from build123d import *

# Parameters (mm, degrees)
SKETCH1_W           = 230
SKETCH1_H           = 150
BOSS_EXTRUDE1_DEPTH = 6
SKETCH2_W           = 11.4
SKETCH2_H           = 3
SKETCH2_H_2         = 3.2
CUT_EXTRUDE1_DEPTH  = 26
SKETCH3_R           = 2.1
CUT_EXTRUDE2_DEPTH  = 26
SKETCH4_R           = 1.6
CUT_EXTRUDE3_DEPTH  = 26
SKETCH5_R           = 1.175
CUT_EXTRUDE4_DEPTH  = 26
SKETCH6_R           = 1.175
CUT_EXTRUDE5_DEPTH  = 26
SKETCH7_W           = 8
SKETCH7_H           = 12
CUT_EXTRUDE6_DEPTH  = 26
FILLET1_R           = 40
SKETCH8_R           = 1.65
CUT_EXTRUDE7_DEPTH  = 26
SKETCH9_R           = 1.6
CUT_EXTRUDE8_DEPTH  = 10
SKETCH10_R          = 1.7
CUT_EXTRUDE9_DEPTH  = 10
SKETCH12_W          = 20
SKETCH12_H          = 6
SKETCH12_W_2        = 6
SKETCH12_H_2        = 20
CUT_EXTRUDE10_DEPTH = 10


with BuildPart() as part:
    # Sketch1 → Boss-Extrude1 (new body)
    with BuildSketch(Plane(origin=(0, 0, 0), x_dir=(1, 0, 0), z_dir=(0, 1, 0))):
        Rectangle(SKETCH1_W, SKETCH1_H)
    extrude(amount=BOSS_EXTRUDE1_DEPTH)

    # Sketch2 → Cut-Extrude1 (cut)
    with BuildSketch(Plane(origin=(0, 6, 0), x_dir=(1, 0, 0), z_dir=(0, 1, 0))):
        with Locations((25, -73.5)):
            Rectangle(SKETCH2_W, SKETCH2_H)
        with Locations((25, -51.4)):
            Rectangle(SKETCH2_W, SKETCH2_H_2)
    cut_extrude1 = extrude(amount=-CUT_EXTRUDE1_DEPTH, mode=Mode.SUBTRACT)

    # Mirror1: Cut-Extrude1 across plane
    add(cut_extrude1.mirror(Plane.XY), mode=Mode.SUBTRACT)

    # Sketch3 → Cut-Extrude2 (cut)
    with BuildSketch(Plane(origin=(0, 6, 0), x_dir=(1, 0, 0), z_dir=(0, 1, 0))):
        with Locations(Location((-25, -12, 0), (0, 0, 270))):
            Circle(SKETCH3_R)
        with Locations(Location((-25, 12, 0), (0, 0, 270))):
            Circle(SKETCH3_R)
        with Locations(Location((-55, 12, 0), (0, 0, 270))):
            Circle(SKETCH3_R)
        with Locations(Location((-55, -12, 0), (0, 0, 270))):
            Circle(SKETCH3_R)
    extrude(amount=-CUT_EXTRUDE2_DEPTH, mode=Mode.SUBTRACT)

    # Sketch4 → Cut-Extrude3 (cut)
    with BuildSketch(Plane(origin=(0, 6, 0), x_dir=(1, 0, 0), z_dir=(0, 1, 0))):
        with Locations(Location((-75, 0, 0), (0, 0, 270))):
            Circle(SKETCH4_R)
        with Locations(Location((-75, 15, 0), (0, 0, 270))):
            Circle(SKETCH4_R)
        with Locations(Location((-75, 30, 0), (0, 0, 270))):
            Circle(SKETCH4_R)
    cut_extrude3 = extrude(amount=-CUT_EXTRUDE3_DEPTH, mode=Mode.SUBTRACT)

    # Mirror2: Cut-Extrude3 across plane
    add(cut_extrude3.mirror(Plane.XY), mode=Mode.SUBTRACT)

    # Sketch5 → Cut-Extrude4 (cut)
    with BuildSketch(Plane(origin=(0, 6, 0), x_dir=(1, 0, 0), z_dir=(0, 1, 0))):
        with Locations(Location((-110, 7.5, 0), (0, 0, 270))):
            Circle(SKETCH5_R)
        with Locations(Location((-110, -7.5, 0), (0, 0, 270))):
            Circle(SKETCH5_R)
    extrude(amount=-CUT_EXTRUDE4_DEPTH, mode=Mode.SUBTRACT)

    # Sketch6 → Cut-Extrude5 (cut)
    with BuildSketch(Plane(origin=(0, 6, 0), x_dir=(1, 0, 0), z_dir=(0, 1, 0))):
        with Locations(Location((-110, 3, 0), (0, 0, 270))):
            Circle(SKETCH6_R)
        with Locations(Location((-110, 18, 0), (0, 0, 270))):
            Circle(SKETCH6_R)
    cut_extrude5 = extrude(amount=-CUT_EXTRUDE5_DEPTH, mode=Mode.SUBTRACT)

    # Mirror3: Cut-Extrude5 across plane
    add(cut_extrude5.mirror(Plane.XY), mode=Mode.SUBTRACT)

    # Sketch7 → Cut-Extrude6 (cut)
    with BuildSketch(Plane(origin=(0, 6, 0), x_dir=(1, 0, 0), z_dir=(0, 1, 0))):
        with Locations((-71, 48.5)):
            Rectangle(SKETCH7_W, SKETCH7_H)
    cut_extrude6 = extrude(amount=-CUT_EXTRUDE6_DEPTH, mode=Mode.SUBTRACT)

    # Mirror4: Cut-Extrude6 across plane
    add(cut_extrude6.mirror(Plane.XY), mode=Mode.SUBTRACT)

    # Fillet1
    fillet1_edges = [part.edges().sort_by_distance(p)[0] for p in [
        (-115, 3, 75),
        (-115, 3, -75),
    ]]
    fillet(fillet1_edges, radius=FILLET1_R)

    # Sketch8 → Cut-Extrude7 (cut)
    with BuildSketch(Plane(origin=(0, 6, 0), x_dir=(1, 0, 0), z_dir=(0, 1, 0))):
        with Locations(Location((-49.5, 63.212121212, 0), (0, 0, 270))):
            Circle(SKETCH8_R)
        with Locations(Location((-49.5, -63.212121212, 0), (0, 0, 270))):
            Circle(SKETCH8_R)
        with Locations(Location((99.5, -63.212121212, 0), (0, 0, 270))):
            Circle(SKETCH8_R)
        with Locations(Location((99.5, 63.212121212, 0), (0, 0, 270))):
            Circle(SKETCH8_R)
    extrude(amount=-CUT_EXTRUDE7_DEPTH, mode=Mode.SUBTRACT)

    # Sketch9 → Cut-Extrude8 (cut)
    with BuildSketch(Plane(origin=(0, 6, 0), x_dir=(1, 0, 0), z_dir=(0, 1, 0))):
        with Locations(Location((-110, -13, 0), (0, 0, 270))):
            Circle(SKETCH9_R)
    cut_extrude8 = extrude(amount=-CUT_EXTRUDE8_DEPTH, mode=Mode.SUBTRACT)

    # Mirror5: Cut-Extrude8 across plane
    add(cut_extrude8.mirror(Plane.XY), mode=Mode.SUBTRACT)

    # Sketch10 → Cut-Extrude9 (cut)
    with BuildSketch(Plane(origin=(0, 6, 0), x_dir=(1, 0, 0), z_dir=(0, 1, 0))):
        with Locations(Location((58.5, 21.5, 0), (0, 0, 270))):
            Circle(SKETCH10_R)
        with Locations(Location((95.5, 21.5, 0), (0, 0, 270))):
            Circle(SKETCH10_R)
        with Locations(Location((95.5, 58.5, 0), (0, 0, 270))):
            Circle(SKETCH10_R)
        with Locations(Location((58.5, 58.5, 0), (0, 0, 270))):
            Circle(SKETCH10_R)
        with Locations(Location((61, -2.75, 0), (0, 0, 270))):
            Circle(SKETCH10_R)
        with Locations(Location((93, -2.75, 0), (0, 0, 270))):
            Circle(SKETCH10_R)
        with Locations(Location((61, -57.25, 0), (0, 0, 270))):
            Circle(SKETCH10_R)
        with Locations(Location((93, -57.25, 0), (0, 0, 270))):
            Circle(SKETCH10_R)
    extrude(amount=-CUT_EXTRUDE9_DEPTH, mode=Mode.SUBTRACT)

    # Sketch12 → Cut-Extrude10 (cut)
    with BuildSketch(Plane(origin=(0, 6, 0), x_dir=(1, 0, 0), z_dir=(0, 1, 0))):
        with Locations((78.5, 65.605966129)):
            Rectangle(SKETCH12_W, SKETCH12_H)
        with Locations((102.815499503, 38.5)):
            Rectangle(SKETCH12_W_2, SKETCH12_H_2)
    cut_extrude10 = extrude(amount=-CUT_EXTRUDE10_DEPTH, mode=Mode.SUBTRACT)

    # Mirror6: Cut-Extrude10 across plane
    add(cut_extrude10.mirror(Plane.XY), mode=Mode.SUBTRACT)


solid = part.part
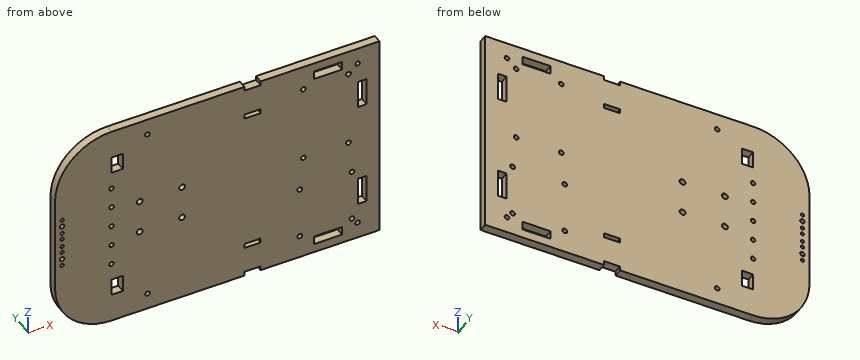
Could you check a few things on this model? Use its own coordinates, in mm. Give positions to 0.01 mm unless a question says otherwise; leave off trailing zeros. Answer as CSV lines item,"result". Start each with the question number.
(1) Please list where these lines run through material, in increasing order: line 1 (X direction, y = 1.5, z = -21.5); line 2 (X direction, y = 4.2, z = 2.75); line 3 (X direction, y = 3.1, z = -30).
(2) If we section it at A-A, the plane y = 4.25: Give the number of separate pieces and of enclosed holes in the cut face, and give its area (3 significant figures).
(3) I'm going to push flat-ended pins straight in: pin 1 Ø1 at (y, z) = (5, -57.5) entering from -X; pin 2 Ø1 at (y, z) = (4, 51) entering from -X; pin 3 Ø1.6 at (y, z) = (3, -50.5) entering from -X. Where does each tip first touch, or does it pass through?
Answer list:
1,line 1,"-115 to 56.8, 60.2 to 93.8, 97.2 to 115"
1,line 2,"-115 to -111.15, -108.85 to 59.3, 62.7 to 91.3, 94.7 to 115"
1,line 3,"-115 to -76.6, -73.4 to 99.82, 105.82 to 115"
2,separate pieces,"1"
2,enclosed holes,"37"
2,area,"32,800 mm^2"
3,pin 1,"x = -108.41"
3,pin 2,"x = -111.87"
3,pin 3,"x = -112.2"
